```python
from build123d import *

# Parameters (mm, degrees)
SKETCH1_W                       = 31.4
SKETCH1_H                       = 31.4
SKETCH1_R                       = 10.25
BOSS_EXTRUDE1_DEPTH             = 40
SKETCH2_R                       = 1.5
CUT_EXTRUDE1_DEPTH              = 40
M4_TAPPED_HOLE1_D               = 3.3
M4_TAPPED_HOLE1_DEPTH           = 10.1
M4_TAPPED_HOLE1_TIP             = 0.991420021
M4_TAPPED_HOLE1_ON_FACE_2_D     = 3.3
M4_TAPPED_HOLE1_ON_FACE_2_DEPTH = 10.1
M4_TAPPED_HOLE1_ON_FACE_2_TIP   = 0.991420021
SKETCH5_R                       = 1.5
CUT_EXTRUDE2_DEPTH              = 40
M4_TAPPED_HOLE2_D               = 3.3
M4_TAPPED_HOLE2_DEPTH           = 10.1
M4_TAPPED_HOLE2_TIP             = 0.991420021
M4_TAPPED_HOLE2_ON_FACE_2_D     = 3.3
M4_TAPPED_HOLE2_ON_FACE_2_DEPTH = 10.1
M4_TAPPED_HOLE2_ON_FACE_2_TIP   = 0.991420021
SKETCH8_R                       = 1.5
CUT_EXTRUDE3_DEPTH              = 30
M4_TAPPED_HOLE3_D               = 3.3
M4_TAPPED_HOLE3_DEPTH           = 52.1
M4_TAPPED_HOLE3_TIP             = 0.991420021
SKETCH10_W                      = 31.4
SKETCH10_H                      = 20
CUT_EXTRUDE4_DEPTH              = 54.220766787


with BuildPart() as part:
    # Sketch1 → Boss-Extrude1 (new body)
    with BuildSketch(Plane(origin=(0, 0, 0), x_dir=(1, 0, 0), z_dir=(0, 1, 0))):
        Rectangle(SKETCH1_W, SKETCH1_H)
        with Locations(Location((0, 0, 0), (0, 0, 270))):
            Circle(SKETCH1_R, mode=Mode.SUBTRACT)
    extrude(amount=BOSS_EXTRUDE1_DEPTH)

    # Sketch2 → Cut-Extrude1 (cut)
    with BuildSketch(Plane(origin=(15.7, 0, 0), x_dir=(0, 0, -1), z_dir=(1, 0, 0))):
        with Locations((0, 30)):
            Circle(SKETCH2_R)
        with Locations((0, 10)):
            Circle(SKETCH2_R)
    extrude(amount=-CUT_EXTRUDE1_DEPTH, mode=Mode.SUBTRACT)

    # M4 Tapped Hole1
    with Locations(Plane(origin=(-15.7, 10, 0), x_dir=(0, 0, -1), z_dir=(-1, 0, 0))):
        with Locations((0, 0), (0, -20)):
            Hole(M4_TAPPED_HOLE1_D / 2, depth=M4_TAPPED_HOLE1_DEPTH)
            with Locations((0, 0, -(M4_TAPPED_HOLE1_DEPTH + M4_TAPPED_HOLE1_TIP / 2))):  # 118° drill point
                Cone(0, M4_TAPPED_HOLE1_D / 2, M4_TAPPED_HOLE1_TIP, mode=Mode.SUBTRACT)

    # M4 Tapped Hole1 on face 2
    with Locations(Plane(origin=(15.7, 30, 0), x_dir=(0, 0, -1), z_dir=(-1, 0, 0))):
        with Locations((0, 0), (0, 20)):
            Hole(M4_TAPPED_HOLE1_ON_FACE_2_D / 2, depth=M4_TAPPED_HOLE1_ON_FACE_2_DEPTH)
            with Locations((0, 0, -(M4_TAPPED_HOLE1_ON_FACE_2_DEPTH + M4_TAPPED_HOLE1_ON_FACE_2_TIP / 2))):  # 118° drill point
                Cone(0, M4_TAPPED_HOLE1_ON_FACE_2_D / 2, M4_TAPPED_HOLE1_ON_FACE_2_TIP, mode=Mode.SUBTRACT)

    # Sketch5 → Cut-Extrude2 (cut)
    with BuildSketch(Plane.XY.offset(15.7)):
        with Locations((0, 30)):
            Circle(SKETCH5_R)
        with Locations((0, 10)):
            Circle(SKETCH5_R)
    extrude(amount=-CUT_EXTRUDE2_DEPTH, mode=Mode.SUBTRACT)

    # M4 Tapped Hole2
    with Locations(Plane(origin=(0, 30, 15.7), x_dir=(1, 0, 0), z_dir=(0, 0, 1))):
        with Locations((0, 0), (0, -20)):
            Hole(M4_TAPPED_HOLE2_D / 2, depth=M4_TAPPED_HOLE2_DEPTH)
            with Locations((0, 0, -(M4_TAPPED_HOLE2_DEPTH + M4_TAPPED_HOLE2_TIP / 2))):  # 118° drill point
                Cone(0, M4_TAPPED_HOLE2_D / 2, M4_TAPPED_HOLE2_TIP, mode=Mode.SUBTRACT)

    # M4 Tapped Hole2 on face 2
    with Locations(Plane(origin=(0, 30, -15.7), x_dir=(1, 0, 0), z_dir=(0, 0, 1))):
        with Locations((0, 0), (0, -20)):
            Hole(M4_TAPPED_HOLE2_ON_FACE_2_D / 2, depth=M4_TAPPED_HOLE2_ON_FACE_2_DEPTH)
            with Locations((0, 0, -(M4_TAPPED_HOLE2_ON_FACE_2_DEPTH + M4_TAPPED_HOLE2_ON_FACE_2_TIP / 2))):  # 118° drill point
                Cone(0, M4_TAPPED_HOLE2_ON_FACE_2_D / 2, M4_TAPPED_HOLE2_ON_FACE_2_TIP, mode=Mode.SUBTRACT)

    # Sketch8 → Cut-Extrude3 (cut)
    with BuildSketch(Plane.XZ):
        with Locations(Location((-10.7, 10.7, 0), (0, 0, 270))):
            Circle(SKETCH8_R)
        with Locations(Location((10.7, 10.7, 0), (0, 0, 90))):
            Circle(SKETCH8_R)
        with Locations(Location((10.7, -10.7, 0), (0, 0, 270))):
            Circle(SKETCH8_R)
        with Locations(Location((-10.7, -10.7, 0), (0, 0, 90))):
            Circle(SKETCH8_R)
    extrude(amount=-CUT_EXTRUDE3_DEPTH, mode=Mode.SUBTRACT)

    # M4 Tapped Hole3
    with Locations(Plane(origin=(-10.7, 0, 10.7), x_dir=(0, 0, -1), z_dir=(0, -1, 0))):
        with Locations((0, 0), (0, 21.4), (21.4, 21.4), (21.4, 0)):
            Hole(M4_TAPPED_HOLE3_D / 2, depth=M4_TAPPED_HOLE3_DEPTH)
            with Locations((0, 0, -(M4_TAPPED_HOLE3_DEPTH + M4_TAPPED_HOLE3_TIP / 2))):  # 118° drill point
                Cone(0, M4_TAPPED_HOLE3_D / 2, M4_TAPPED_HOLE3_TIP, mode=Mode.SUBTRACT)

    # Sketch10 → Cut-Extrude4 (cut, through all)
    with BuildSketch(Plane.XY.offset(15.7)):
        with Locations((0, 30)):
            Rectangle(SKETCH10_W, SKETCH10_H)
    extrude(amount=-CUT_EXTRUDE4_DEPTH, mode=Mode.SUBTRACT)


solid = part.part
```
Work out the finished part from the listing and answer in its coordinate system (mm). Coordinates: 2 decimals unless noted, no trailing zeros. Order: outer loops, then holes, each group sorted by start corner. A loop starts at its lowest first (then second) coordinate and runs counter-clockwise, first axis right, second up. Notation, with made-up numbers: (71.5, 8) - (104.5, 8) arc R31 ccw to (104.5, 32) - close; hole circle Ø9 at (7.5, 65.5). An arc over 180 degrees is marked (long way). Answer as a JSON object with one key per item and string values.
1. The mould has two halves that part along X. Classify faces 1 (the face through (-15.7, 12, 0)), 2 (the face through (10.068, 10.14, -9.176)), 3 (the face through (-12.9, 11.6, -0.4)), 4 (the face through (15.7, 12, 0)): +X half, -X half, draft (parallel to the pull), parting line (faces both ways), or undercut.
Output values:
{"face 1": "-X half", "face 2": "undercut", "face 3": "draft", "face 4": "+X half"}
2. Find section D-D on z = 0. Determine the outline of the cut face in (x, y).
Output values:
{"outline": "(-15.7, 0) - (-10.25, 0) - (-10.25, 8.35) - (-15.7, 8.35) - close; (-15.7, 11.65) - (-10.25, 11.65) - (-10.25, 20) - (-15.7, 20) - close; (10.25, 0) - (15.7, 0) - (15.7, 8.35) - (10.25, 8.35) - close; (10.25, 11.65) - (15.7, 11.65) - (15.7, 20) - (10.25, 20) - close"}
3. Consider line 1 (X direction, y = 14.25, z = 10.7); line 2 (Y direction, x = 12.1, z = 0); line 3 (X direction, y = 16.5, z = 12). Determine where each line is inside the solid, lowest interval first.
Output values:
{"line 1": "x = -15.7 to -12.35, -9.05 to 9.05, 12.35 to 15.7", "line 2": "y = 0 to 8.35, 11.65 to 20", "line 3": "x = -15.7 to -11.72, -9.68 to 9.68, 11.72 to 15.7"}
4. Find section A-A on x = -10.7. Determine the outline of the cut face in (y, z), plus the area to 3 significant figures.
Output values:
{"outline": "(0, -15.7) - (20, -15.7) - (20, -12.35) - (0, -12.35) - close; (0, -9.05) - (20, -9.05) - (20, 9.05) - (0, 9.05) - close; (0, 12.35) - (20, 12.35) - (20, 15.7) - (0, 15.7) - close; hole circle Ø3.3 at (10, 0)", "area": "487 mm²"}
5. Find section C-C on x = 0. Determine the outline of the cut face in (y, z), plus the area to 3 significant figures.
Output values:
{"outline": "(0, -15.7) - (8.35, -15.7) - (8.35, -10.25) - (0, -10.25) - close; (0, 10.25) - (8.35, 10.25) - (8.35, 15.7) - (0, 15.7) - close; (11.65, -15.7) - (20, -15.7) - (20, -10.25) - (11.65, -10.25) - close; (11.65, 10.25) - (20, 10.25) - (20, 15.7) - (11.65, 15.7) - close", "area": "182 mm²"}
6. Find section B-B on z = -10.7. Determine the outline of the cut face in (x, y).
Output values:
{"outline": "(-15.7, 0) - (-12.35, 0) - (-12.35, 20) - (-15.7, 20) - close; (-9.05, 0) - (9.05, 0) - (9.05, 20) - (-9.05, 20) - close; (12.35, 0) - (15.7, 0) - (15.7, 20) - (12.35, 20) - close; hole circle Ø3.3 at (0, 10)"}
